Verification items for the finished model (mm, model axes). Face numbers are marked on the shaded views. A direction names the side the tool comes from. Round coordinates to 2 decimals unless told otherwise and drop trailing zeros. Write each loop counter-clockwise with the first axis right and the second up, starting at its lowest first coordinate (ties: lowest second). Pieces come first, ordered by that corner, then holes. Notation, with made-up numbers: M 32.5,76.25 L 73.5,76.25 A24 ccw 73.5,101.25 Z; hole C 34.25,20 d6. An arc over 180 degrees is marked long. One line per question, with ' | ' between items.
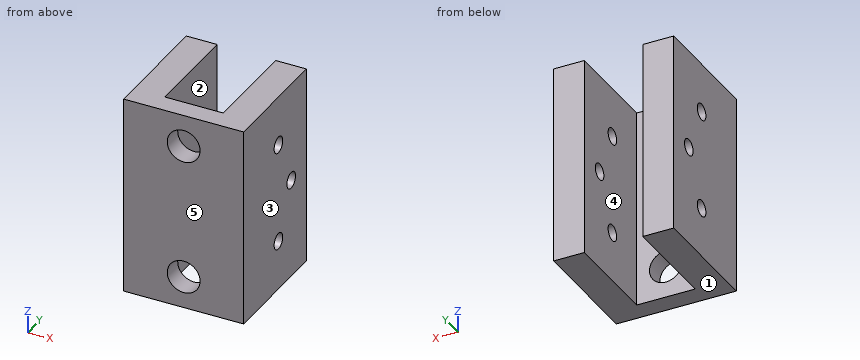
from build123d import *

# Parameters (mm, degrees)
SKETCH1_W           = 30
SKETCH1_H           = 50
SKETCH1_R           = 4.1
BOSS_EXTRUDE1_DEPTH = 5
BOSS_EXTRUDE2_DEPTH = 25
SKETCH4_R           = 2.05
CUT_EXTRUDE1_DEPTH  = 50.244289009
SKETCH5_W           = 14.6
SKETCH5_H           = 50
CUT_EXTRUDE2_DEPTH  = 25


with BuildPart() as part:
    # Sketch1 → Boss-Extrude1 (new body)
    with BuildSketch(Plane(origin=(0, 0, 0), x_dir=(1, 0, 0), z_dir=(0, 1, 0))):
        Rectangle(SKETCH1_W, SKETCH1_H)
        with Locations(Location((0, 17, 0), (0, 0, 270))):
            Circle(SKETCH1_R, mode=Mode.SUBTRACT)
        with Locations(Location((0, -17, 0), (0, 0, 270))):
            Circle(SKETCH1_R, mode=Mode.SUBTRACT)
    extrude(amount=BOSS_EXTRUDE1_DEPTH)

    # Sketch2 → Boss-Extrude2 (add)
    with BuildSketch(Plane(origin=(0, 5, 0), x_dir=(1, 0, 0), z_dir=(0, 1, 0))):
        Polygon((-7.25, -9.75), (7.25, -9.75), (7.25, -25), (15, -25), (15, 25), (7.25, 25), (7.25, 9.75), (-7.25, 9.75), (-7.25, 25), (-15, 25), (-15, -25), (-7.25, -25), align=None)
    extrude(amount=BOSS_EXTRUDE2_DEPTH)

    # Sketch4 → Cut-Extrude1 (cut, through all)
    with BuildSketch(Plane(origin=(15, 0, 0), x_dir=(0, 0, -1), z_dir=(1, 0, 0))):
        with Locations((-12.54526483, 16.63)):
            Circle(SKETCH4_R)
        with Locations((12.54526483, 16.63)):
            Circle(SKETCH4_R)
        with Locations((0, 22.755)):
            Circle(SKETCH4_R)
    extrude(amount=-CUT_EXTRUDE1_DEPTH, mode=Mode.SUBTRACT)

    # Sketch5 → Cut-Extrude2 (cut)
    with BuildSketch(Plane(origin=(0, 30, 0), x_dir=(1, 0, 0), z_dir=(0, 1, 0))):
        Rectangle(SKETCH5_W, SKETCH5_H)
    extrude(amount=-CUT_EXTRUDE2_DEPTH, mode=Mode.SUBTRACT)


solid = part.part
1. Section check D-D, the plane x = 0. Record the cut outline in (y, z), then the cut area to 3 significant figures.
Results:
outline: M 0,-25 L 5,-25 L 5,-21.1 L 0,-21.1 Z; M 0,-12.9 L 5,-12.9 L 5,12.9 L 0,12.9 Z; M 0,21.1 L 5,21.1 L 5,25 L 0,25 Z | area: 168 mm2
2. Section check A-A, the plane z = 0. Record the cut outline in (x, y) (3 decimals), then the cut area to 3 significant figures.
Results:
outline: M -15,0 L 15,0 L 15,20.705 L 7.3,20.705 L 7.3,5 L -7.3,5 L -7.3,20.705 L -15,20.705 Z; M -15,24.805 L -7.3,24.805 L -7.3,30 L -15,30 Z; M 7.3,24.805 L 15,24.805 L 15,30 L 7.3,30 Z | area: 472 mm2
3. Tool access check on the marked faces 4 and 5. Record the directions out of +Z, -Z, +X, -X, +Y, -Y that give a thin tool (end or side, any length) a straight path to the whole face; none if there is none.
Results:
face 4: +Z, -Z, +Y | face 5: +Z, -Z, +X, -X, -Y
4. Section check C-C, the plane z = 17. Record the cut outline in (x, y).
Results:
outline: M -15,0 L -4.1,0 L -4.1,5 L -7.3,5 L -7.3,30 L -15,30 Z; M 4.1,0 L 15,0 L 15,30 L 7.3,30 L 7.3,5 L 4.1,5 Z
5. Thickness scan on line 1 (X direction, y = 16, z = -3); line 2 (Z direction, x = 10.25, y = 18); line 3 (Z direction, x = 2, y = 2.25). Record the ranges inside material, lowest first.
Results:
line 1: x = -15 to -7.3, 7.3 to 15 | line 2: z = -25 to -14.07, -11.02 to 11.02, 14.07 to 25 | line 3: z = -25 to -20.58, -13.42 to 13.42, 20.58 to 25
6. Section check B-B, the plane y = 7. Record the cut outline in (x, z).
Results:
outline: M -15,-25 L -7.3,-25 L -7.3,25 L -15,25 Z; M 7.3,-25 L 15,-25 L 15,25 L 7.3,25 Z
7. Go/stop test with flat-tipped pins: P1, Ø2.5, axis at y = 16.63, z = -12.55, coming from the +X side; P2, Ø11.5, axis at x = 1.5, z = 8, coming from the +Y side. Record where each tip stops, or that it passes through.
Results:
P1: passes through | P2: stops at y = 5
8. Mould release check, pull along X, two halves, no side actions. Record for the marked faces 1, 2 and 3: pulls with the +X half, pulls with the -X half, needs draft (parallel to the pull), parting line crosses it, or undercut.
Results:
face 1: needs draft | face 2: undercut | face 3: pulls with the +X half
